Geometry check sheet. Reference: the model listing, model coordinates, mm. A direction names the side the tool comes from. Coordinates: 2 decimals unless noted, no trailing zeros. Write each loop counter-clockwise with the first axis right and the second up, starting at its lowest first coordinate (ties: lowest second). Pieces come first, ordered by that corner, then holes.
from build123d import *

# Parameters (mm, degrees)
F1_DEPTH = 7
F2_SIZE  = 1


with BuildPart() as f1:
    # F0 (on Top) → F1 (new body)
    with BuildSketch(Plane.XY):
        Polygon((-0.9, -5), (-0.9, 0), (-2.8, 0), (-2.8, -2.8), (-2.8, -5), align=None)
        Polygon((-2.8, 0), (-0.9, 0), (0.9, 0), (2.8, 0), (4.05, 0), (4.05, -2), (5.55, -2), (5.55, 2), (0, 2), (-5.55, 2), (-5.55, -2), (-4.05, -2), (-4.05, 0), align=None)
        Polygon((2.8, 0), (0.9, 0), (0.9, -5), (2.8, -5), (2.8, -2.8), align=None)
        Polygon((-2.8, -5), (-2.8, -2.8), (-3.5, -3.5), (-3.5, -4.3), align=None)
        Polygon((2.8, -2.8), (2.8, -5), (3.5, -4.3), (3.5, -3.5), align=None)
    extrude(amount=F1_DEPTH)

    # F2
    f2_edges = [f1.edges().sort_by_distance(p)[0] for p in [
        (-5.55, 2, 3.5),
        (5.55, 2, 3.5),
    ]]
    chamfer(f2_edges, length=F2_SIZE)


solid = f1.part
1. Sectioned sample at C-C, the plane z = 5. Record the boundary of the cut face in (x, y), and give its area (3 significant figures).
Computed values:
outline: (-5.55, -2) - (-4.05, -2) - (-4.05, 0) - (-2.8, 0) - (-2.8, -2.8) - (-3.5, -3.5) - (-3.5, -4.3) - (-2.8, -5) - (-0.9, -5) - (-0.9, 0) - (0.9, 0) - (0.9, -5) - (2.8, -5) - (3.5, -4.3) - (3.5, -3.5) - (2.8, -2.8) - (2.8, 0) - (4.05, 0) - (4.05, -2) - (5.55, -2) - (5.55, 1) - (4.55, 2) - (-4.55, 2) - (-5.55, 1) - close
area: 48.3 mm2
2. Draft check along Y on faces 4 (the flat face through (2.8, -1, 3)), 5 (the flat face through (1.2, -0.7, 0)), 6 (the flat face through (-2, -5, 3)), 7 (the flat face through (3, 0, 3)). Enter one of: released by +Y, released by -Y, zero draft, split by the parting line, or undercut.
Computed values:
face 4: undercut
face 5: zero draft
face 6: released by -Y
face 7: undercut
3. Access from +Z, -Z, +X, -X, +Y, -Y to the whole of each face (thin tool, end or side, straight path). Record for faces 1 (the flat face through (-3, 0, 3)), 2 (the flat face through (5, -2, 3)), 3 (the flat face through (0.9, -2, 3)).
Computed values:
face 1: +Z, -Z
face 2: +Z, -Z, +X, -Y
face 3: +Z, -Z, -Y
4. Sectioned sample at B-B, the plane y = -1. Record the boundary of the cut face in (x, z).
Computed values:
outline: (-5.55, 0) - (-4.05, 0) - (-4.05, 7) - (-5.55, 7) - close; (-2.8, 0) - (-0.9, 0) - (-0.9, 7) - (-2.8, 7) - close; (0.9, 0) - (2.8, 0) - (2.8, 7) - (0.9, 7) - close; (4.05, 0) - (5.55, 0) - (5.55, 7) - (4.05, 7) - close
5. Sectioned sample at A-A, the plane y = -2.5. Record the boundary of the cut face in (x, z).
Computed values:
outline: (-2.8, 0) - (-0.9, 0) - (-0.9, 7) - (-2.8, 7) - close; (0.9, 0) - (2.8, 0) - (2.8, 7) - (0.9, 7) - close
6. Gauge pin test, flat ends, axial feed: pin 1 Ø1 at (x, z) = (0, 3.5) entering from -Y; pin 2 Ø0.9 at (y, z) = (-4, 2.5) entering from +X; pin 3 Ø4 at (y, z) = (-3.5, 2.5) entering from -X; pin 4 Ø0.8 at (x, z) = (5, 4.5) entering from -Y. Record the tip position at first contact, or that the pin passes through.
Computed values:
pin 1: stops at y = 0
pin 2: stops at x = 3.5
pin 3: stops at x = -5.55
pin 4: stops at y = -2
7. Sectioned sample at D-D, the plane x = 0.5. Record the boundary of the cut face in (y, z).
Computed values:
outline: (0, 0) - (2, 0) - (2, 7) - (0, 7) - close
8. Thickness scan on line 1 along X through (y, z) = (-1.5, 5.25); line 2 along X through (y, z) = (-2.5, 6); line 3 along Y through (x, z) = (0.25, 1.5). Record the ranges inside material, lowest first.
Computed values:
line 1: x = -5.55 to -4.05, -2.8 to -0.9, 0.9 to 2.8, 4.05 to 5.55
line 2: x = -2.8 to -0.9, 0.9 to 2.8
line 3: y = 0 to 2
